Read the model definition and answer for the solid it produces. Units are mm, in the model's axes. A direction names the side the tool comes from. Coordinates: 2 decimals unless noted, no trailing zeros. Order: outer loops, then holes, each group sorted by start corner. A loop starts at its lowest first (then second) coordinate and runs counter-clockwise, first axis right, second up.
```python
from build123d import *

# Parameters (mm, degrees)
SKETCH_2_R      = 2.75
EXTRUDE_1_DEPTH = 3
SKETCH_3_R      = 1.5
EXTRUDE_2_DEPTH = 15
FILLET_1_R      = 0.5


with BuildPart() as part:
    # ｽｹｯﾁ2 → ﾎﾞｽ - 押し出し1 (new body)
    with BuildSketch(Plane.XY):
        Circle(SKETCH_2_R)
    extrude(amount=EXTRUDE_1_DEPTH)

    # ｽｹｯﾁ3 → ﾎﾞｽ - 押し出し2 (add)
    with BuildSketch(Plane.XY.offset(3)):
        Circle(SKETCH_3_R)
    extrude(amount=EXTRUDE_2_DEPTH)

    # ﾌｨﾚｯﾄ1
    fillet_1_edges = [part.edges().sort_by_distance(p)[0] for p in [
        (-2.75, 0, 0),
    ]]
    fillet(fillet_1_edges, radius=FILLET_1_R)


solid = part.part
```
1) A cutting plane is placed at A-A, the plane x = 0. Determine the outline of the cut face in (y, z), and give its area (3 significant figures).
A:
outline: (-2.75, 0.5) arc R0.5 ccw to (-2.25, 0) - (2.25, 0) arc R0.5 ccw to (2.75, 0.5) - (2.75, 3) - (1.5, 3) - (1.5, 18) - (-1.5, 18) - (-1.5, 3) - (-2.75, 3) - close
area: 61.4 mm2
2) Which of the six approach directions +Z, -Z, +X, -X, +Y, -Y give full straight-line access (tool end or side, diameter ignored) to faces 1 (the flat face through (0, 0, 18)), 2 (the flat face through (1.2, -1.2, 3))?
A:
face 1: +Z, +X, -X, +Y, -Y
face 2: +Z
3) Flat-ended cylindrical pins translate along their axes: pin 1 Ø1.5 at (y, z) = (-2, 5.5) entering from +X; pin 2 Ø3 at (y, z) = (2, 14) entering from -X; pin 3 Ø1 at (x, z) = (1, 13.5) entering from +Y. Find the tip coordinate at first contact, or state that the pin passes through.
A:
pin 1: stops at x = 0.83
pin 2: stops at x = -1.41
pin 3: stops at y = 1.41
4) A cutting plane is placed at D-D, the plane z = 14.25. Determine the outline of the cut face in (x, y).
A:
outline: circle Ø3 at (0, 0)
5) A cutting plane is placed at C-C, the plane z = 2.25. Determine the outline of the cut face in (x, y), and give its area (3 significant figures).
A:
outline: circle Ø5.5 at (0, 0)
area: 23.8 mm2
6) Straight lines are drawn through the part: line 1 (Z direction, x = 0.65, y = -1.6); line 2 (Y direction, x = 0.05, z = 11); line 3 (X direction, y = -0.8, z = 6). For each, find the intervals that lie inside material, in ascending order.
A:
line 1: z = 0 to 3
line 2: y = -1.5 to 1.5
line 3: x = -1.27 to 1.27
